from build123d import *

# Parameters (mm, degrees)
SKETCH1_R               = 50
BOSS_EXTRUDE1_DEPTH     = 140
SKETCH2_W               = 10
SKETCH2_H               = 60
BOSS_EXTRUDE2_START     = 100
SKETCH3_R               = 50
BOSS_EXTRUDE2_DEPTH     = 100
SKETCH4_R               = 169.268161275
BOSS_EXTRUDE3_DEPTH     = 10
FILLET2_R               = 50
CUT_EXTRUDE1_DEPTH      = 278.314660346
CUT_EXTRUDE1_DEPTH_BACK = 278.314660346
SKETCH5_W               = 561.706839888
SKETCH5_H               = 604.768431274
SKETCH6_R               = 20
BOSS_EXTRUDE4_DEPTH     = 116
SKETCH7_W               = 77.5
SKETCH7_H               = 80.450571877


with BuildPart() as part:
    # Sketch1 → Boss-Extrude1 (new body)
    with BuildSketch(Plane(origin=(0, 0, 0), x_dir=(0, 0, -1), z_dir=(1, 0, 0))):
        Circle(SKETCH1_R)
    extrude(amount=BOSS_EXTRUDE1_DEPTH)

    # Sketch2 → Revolve1 (revolve)
    with BuildSketch(Plane(origin=(0, 0, 0), x_dir=(1, 0, 0), z_dir=(0, 1, 0)), mode=Mode.PRIVATE) as revolve1_sk:
        with Locations((15, 30)):
            Rectangle(SKETCH2_W, SKETCH2_H)
        with Locations((125, 30)):
            Rectangle(SKETCH2_W, SKETCH2_H)
    revolve(revolve1_sk.sketch.rotate(Axis((0, 0, 0), (1, 0, 0)), 180), axis=Axis((0, 0, 0), (1, 0, 0)))

    # Sketch3 → Boss-Extrude2 (add)
    with BuildSketch(Plane.ZY.offset(BOSS_EXTRUDE2_START)):
        Circle(SKETCH3_R)
    extrude(amount=-BOSS_EXTRUDE2_DEPTH)

    # Sketch4 → Boss-Extrude3 (add)
    with BuildSketch(Plane.ZY.offset(100)):
        Circle(SKETCH4_R)
    extrude(amount=BOSS_EXTRUDE3_DEPTH)

    # Fillet2
    fillet2_edges = [part.edges().sort_by_distance(p)[0] for p in [
        (-100, 0, -50),
    ]]
    fillet(fillet2_edges, radius=FILLET2_R)

    # Sketch5 → Cut-Extrude1 (cut, two sides: drawn at the far end of the back side and taken through both)
    with BuildSketch(Plane(origin=(0, 0, 0), x_dir=(1, 0, 0), z_dir=(0, 1, 0)).offset(-CUT_EXTRUDE1_DEPTH_BACK)):
        with Locations((180.853419944, 0)):
            Rectangle(SKETCH5_W, SKETCH5_H)
    extrude(amount=CUT_EXTRUDE1_DEPTH + CUT_EXTRUDE1_DEPTH_BACK, mode=Mode.SUBTRACT)

    # Sketch6 → Boss-Extrude4 (add)
    with BuildSketch(Plane(origin=(-100, 0, 0), x_dir=(0, 0, -1), z_dir=(1, 0, 0))):
        with Locations(Location((0, 0, 0), (0, 0, 180))):
            Circle(SKETCH6_R)
    extrude(amount=BOSS_EXTRUDE4_DEPTH)

    # Sketch7 → Revolve2 (revolve)
    with BuildSketch(Plane(origin=(0, 0, 0), x_dir=(1, 0, 0), z_dir=(0, 1, 0)), mode=Mode.PRIVATE) as revolve2_sk:
        with Locations((-61.25, 40.225285939)):
            Rectangle(SKETCH7_W, SKETCH7_H)
    revolve(revolve2_sk.sketch.rotate(Axis((-151.154136958, 0, 0), (1, 0, 0)), 180), axis=Axis((-151.154136958, 0, 0), (1, 0, 0)))


solid = part.part
CAD build for the part. Positions are in the model's coordinates, mm. A direction names the side the tool comes from. Coordinates: 2 decimals unless noted, no trailing zeros. Write each loop counter-clockwise with the first axis right and the second up, starting at its lowest first coordinate (ties: lowest second). Pieces come first, ordered by that corner, then holes. Notation, with made-up numbers: (12, 11) - (28, 11) arc R18 cw to (28, 28) - close; hole circle Ø5 at (-37.5, -29.75). An arc over 180 degrees is marked (long way). Use a Markdown table: item, result. Add a question column.
Item 1: Band-saw the part on C-C, the plane x = -31. Give the cut face in (y, z), and give its area (3 significant figures).
Item 2: Band-saw the part on A-A, the plane z = 0. Give the cut face in (x, y).
Item 3: 3-axis set-ups, long thin cutter, end or side, ignore diameter. For faces 1 (the face through (-104.93, 7.442, -169.104)), 2 (the face through (-22.5, 17, -17)): which of +Z, -Z, +X, -X, +Y, -Y reach the whole face in a straight line?
Item 4: Flat gauge pins, fed straight in: pin 1 (1 mm diameter, centred on y = 134, z = 14.5, fed in from +X); pin 2 (10 mm diameter, centred on y = -24, z = -75, fed in from +X); pin 3 (4 mm diameter, centred on x = -40, y = -10.5, fed in from +Z). Where does each tip first touch, or does it go through?
Item 5: Drill centre lines: L1, parallel to X at y = 110.5, z = -101; L2, parallel to X at y = -23.5, z = 37; L3, parallel to Z at x = -94, y = -23. Where is each one in solid material? Low to high. Write a range as from..to.
Item 6: Band-saw the part on D-D, the plane y = -48. Give the cut face in (x, z), and give its area (3 significant figures).
Numbers:
| question | item | result |
|---|---|---|
| 1 | outline | circle Ø160.9 at (0, 0) |
| 1 | area | 20,300 mm2 |
| 2 | outline | (-110, -169.27) - (-100, -169.27) - (-100, -80.45) - (-22.5, -80.45) - (-22.5, -20) - (16, -20) - (16, 20) - (-22.5, 20) - (-22.5, 80.45) - (-100, 80.45) - (-100, 169.27) - (-110, 169.27) - close |
| 3 | face 1 | +X, -X |
| 3 | face 2 | +X |
| 4 | pin 1 | x = -100 |
| 4 | pin 2 | x = -22.5 |
| 4 | pin 3 | z = 80 |
| 5 | L1 | -110..-100 |
| 5 | L2 | -110..-22.5 |
| 5 | L3 | -77.09..77.09 |
| 6 | outline | (-110, -162.32) - (-100, -162.32) - (-100, -64.56) - (-22.5, -64.56) - (-22.5, 64.56) - (-100, 64.56) - (-100, 162.32) - (-110, 162.32) - close |
| 6 | area | 13,300 mm2 |
